Source: CAD feature listing. Evaluate the final solid. Frame: model axes, mm. Face numbers are marked on the shaded views. A direction names the side the tool comes from. Round coordinates to 2 decimals unless told otherwise and drop trailing zeros. Order: outer loops, then holes, each group sorted by start corner. A loop starts at its lowest first (then second) coordinate and runs counter-clockwise, first axis right, second up. Notation, with made-up numbers: (29, -30.75) -> (77, -30.75) arc R12 ccw to (77, -19.75) -> close; hole circle Ø11 at (1, 76.5). An arc over 180 degrees is marked (long way). Answer as CSV lines item,"result".
from build123d import *

# Parameters (mm, degrees)
SKETCH1_W           = 30
SKETCH1_H           = 73
BOSS_EXTRUDE1_DEPTH = 26
SKETCH2_W           = 25
SKETCH2_H           = 16.1
CUT_EXTRUDE1_DEPTH  = 74
SKETCH3_W           = 26
SKETCH3_H           = 24
SKETCH3_H_2         = 16.23422306
CUT_EXTRUDE2_DEPTH  = 5
SKETCH5_W           = 60
SKETCH5_H           = 60
BOSS_EXTRUDE2_DEPTH = 5
FILLET1_R           = 5
SKETCH6_R           = 1.5
CUT_EXTRUDE4_DEPTH  = 5
SKETCH7_R           = 1
CUT_EXTRUDE5_DEPTH  = 4
SKETCH8_W           = 15.5
SKETCH8_H           = 5
CUT_EXTRUDE6_DEPTH  = 42
SKETCH9_W           = 5
SKETCH9_H           = 26
CUT_EXTRUDE7_DEPTH  = 73
SKETCH10_W          = 2
SKETCH10_H          = 8
SKETCH10_H_2        = 7.5
BOSS_EXTRUDE3_DEPTH = 78
SKETCH11_W          = 42
SKETCH11_H          = 0.6
CUT_EXTRUDE8_DEPTH  = 6
SKETCH13_W          = 0.6
SKETCH13_H          = 5
BOSS_EXTRUDE5_DEPTH = 2
SKETCH15_W          = 4
SKETCH15_H          = 16.1
BOSS_EXTRUDE6_DEPTH = 78


with BuildPart() as part:
    # Sketch1 → Boss-Extrude1 (new body)
    with BuildSketch(Plane.XY):
        Rectangle(SKETCH1_W, SKETCH1_H)
    extrude(amount=BOSS_EXTRUDE1_DEPTH)

    # Sketch2 → Cut-Extrude1 (cut, through all)
    with BuildSketch(Plane(origin=(0, 36.5, 0), x_dir=(1, 0, 0), z_dir=(0, 1, 0))):
        with Locations((-0.5, -13.05)):
            Rectangle(SKETCH2_W, SKETCH2_H)
    extrude(amount=-CUT_EXTRUDE1_DEPTH, mode=Mode.SUBTRACT)

    # Sketch3 → Cut-Extrude2 (cut)
    with BuildSketch(Plane.ZY.offset(15)):
        with Locations((13, 21.5)):
            Rectangle(SKETCH3_W, SKETCH3_H)
        with Locations((13, -5.5)):
            Rectangle(SKETCH3_W, SKETCH3_H)
        with Locations((13, -28.61711153)):
            Rectangle(SKETCH3_W, SKETCH3_H_2)
    extrude(amount=-CUT_EXTRUDE2_DEPTH, mode=Mode.SUBTRACT)

    # Sketch5 → Boss-Extrude2 (add)
    with BuildSketch(Plane(origin=(0, -36.5, 0), x_dir=(-1, 0, 0), z_dir=(0, -1, 0))):
        with Locations((0, -13)):
            Rectangle(SKETCH5_W, SKETCH5_H)
    extrude(amount=BOSS_EXTRUDE2_DEPTH)

    # Fillet1
    fillet1_edges = [part.edges().sort_by_distance(p)[0] for p in [
        (30, -39, -17),
        (30, -39, 43),
        (-30, -39, 43),
        (-30, -39, -17),
    ]]
    fillet(fillet1_edges, radius=FILLET1_R)

    # Sketch6 → Cut-Extrude4 (cut)
    with BuildSketch(Plane(origin=(0, -36.5, 0), x_dir=(1, 0, 0), z_dir=(0, 1, 0))):
        with Locations((-24.540514854, 12.671548216)):
            Circle(SKETCH6_R)
        with Locations((24.540514854, 12.671548216)):
            Circle(SKETCH6_R)
        with Locations((-24.540514854, -38.671548216)):
            Circle(SKETCH6_R)
        with Locations((24.540514854, -38.671548216)):
            Circle(SKETCH6_R)
    extrude(amount=-CUT_EXTRUDE4_DEPTH, mode=Mode.SUBTRACT)

    # Sketch7 → Cut-Extrude5 (cut)
    with BuildSketch(Plane(origin=(0, 0, 0), x_dir=(-1, 0, 0), z_dir=(0, 0, -1))):
        with Locations((-7, 31.5)):
            Circle(SKETCH7_R)
        with Locations((-12, 24.5)):
            Circle(SKETCH7_R)
        with Locations((-2, 24.5)):
            Circle(SKETCH7_R)
        with Locations((-7, 18.5)):
            Circle(SKETCH7_R)
    extrude(amount=-CUT_EXTRUDE5_DEPTH, mode=Mode.SUBTRACT)

    # Sketch8 → Cut-Extrude6 (cut)
    with BuildSketch(Plane.ZY.offset(30)):
        with Locations((12.75, -39)):
            Rectangle(SKETCH8_W, SKETCH8_H)
    extrude(amount=-CUT_EXTRUDE6_DEPTH, mode=Mode.SUBTRACT)

    # Sketch9 → Cut-Extrude7 (cut)
    with BuildSketch(Plane(origin=(0, 36.5, 0), x_dir=(1, 0, 0), z_dir=(0, 1, 0))):
        with Locations((-12.5, -13)):
            Rectangle(SKETCH9_W, SKETCH9_H)
    extrude(amount=-CUT_EXTRUDE7_DEPTH, mode=Mode.SUBTRACT)

    # Sketch10 → Boss-Extrude3 (add)
    with BuildSketch(Plane(origin=(0, 36.5, 0), x_dir=(1, 0, 0), z_dir=(0, 1, 0))):
        with Locations((-11, -4)):
            Rectangle(SKETCH10_W, SKETCH10_H)
        with Locations((-11, -22.25)):
            Rectangle(SKETCH10_W, SKETCH10_H_2)
    extrude(amount=-BOSS_EXTRUDE3_DEPTH)

    # Sketch11 → Cut-Extrude8 (cut, through all)
    with BuildSketch(Plane(origin=(0, -36.5, 0), x_dir=(1, 0, 0), z_dir=(0, 1, 0))):
        with Locations((-9, -20.8)):
            Rectangle(SKETCH11_W, SKETCH11_H)
    extrude(amount=-CUT_EXTRUDE8_DEPTH, mode=Mode.SUBTRACT)

    # Sketch13 → Boss-Extrude5 (add)
    with BuildSketch(Plane.ZY.offset(12)):
        with Locations((20.8, -39)):
            Rectangle(SKETCH13_W, SKETCH13_H)
    extrude(amount=-BOSS_EXTRUDE5_DEPTH)

    # Sketch15 → Boss-Extrude6 (add)
    with BuildSketch(Plane(origin=(0, 36.5, 0), x_dir=(1, 0, 0), z_dir=(0, 1, 0))):
        with Locations((4.6, -13.05)):
            Rectangle(SKETCH15_W, SKETCH15_H)
    extrude(amount=-BOSS_EXTRUDE6_DEPTH)


solid = part.part
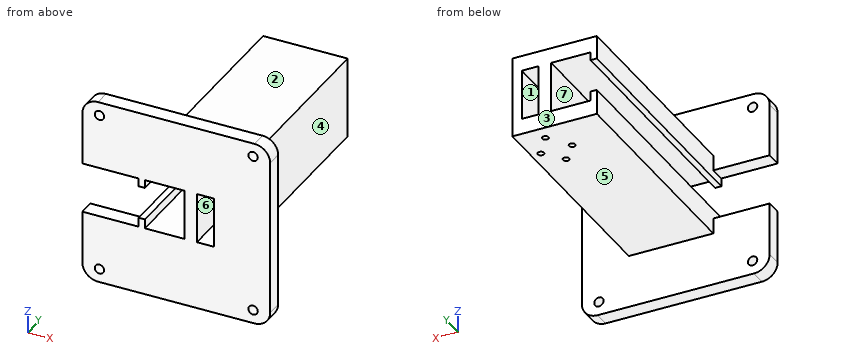
1. Section query C-C on x = -11. Return loops of the section in (y, z).
Results below:
outline,"(-41.5, -17) -> (-36.5, -17) -> (-36.5, 0) -> (36.5, 0) -> (36.5, 8) -> (-41.5, 8) -> close; (-41.5, 18.5) -> (36.5, 18.5) -> (36.5, 26) -> (-36.5, 26) -> (-36.5, 43) -> (-41.5, 43) -> close"
2. Pin query (flat end, axial travel): pin 1 (3 mm diameter, centred on y = -12, z = 26.5, fed in from +X); pin 2 (2 mm diameter, centred on x = 15, y = -17.5, fed in from -Z); pin 3 (5 mm diameter, centred on x = 24.54, z = -12.67, fed in from -Y); pin 4 (1 mm diameter, centred on x = -11, y = 2.5, fed in from +Z). Return the tip coordinate at first contact, or that it passes through.
Results below:
pin 1,"x = 15"
pin 2,"z = 0"
pin 3,"y = -41.5"
pin 4,"z = 26"
3. Section query A-A on z = 16. Return loops of the section in (x, y).
Results below:
outline,"(2.6, -41.5) -> (6.6, -41.5) -> (6.6, 36.5) -> (2.6, 36.5) -> close; (12, -41.5) -> (30, -41.5) -> (30, -36.5) -> (15, -36.5) -> (15, 36.5) -> (12, 36.5) -> close"
4. Reachability of the marked faces 1, 2 and 3 from +Z, -Z, +X, -X, +Y, -Y: full face, straight path, thin tool, end or side. Return the list, or none.
Results below:
face 1,"+Y, -Y"
face 2,"+Z, +X, -X, +Y"
face 3,"+Z, -Z, +X, -X, +Y"
5. Mould query, pull axis Z, two halves, no side actions, for the marked faces 4, 5, 6 and 7. Classes: released by +Z, released by -Z, zero draft, split by the parting line, or undercut.
Results below:
face 4,"zero draft"
face 5,"released by -Z"
face 6,"undercut"
face 7,"undercut"
6. Section query D-D on x = -17.5. Return loops of the section in (y, z), and give its area (4 significant figures).
Results below:
outline,"(-41.5, -17) -> (-36.5, -17) -> (-36.5, 5) -> (-41.5, 5) -> close; (-41.5, 21.1) -> (-36.5, 21.1) -> (-36.5, 43) -> (-41.5, 43) -> close"
area,"219.5 mm2"
7. Section query B-B on y = 18.5. Return loops of the section in (x, z), and give its area (3 significant figures).
Results below:
outline,"(-12, 0) -> (6, 0) -> (6, 4) -> (8, 4) -> (8, 0) -> (15, 0) -> (15, 26) -> (-12, 26) -> (-12, 18.5) -> (-10, 18.5) -> (-10, 21.1) -> (2.6, 21.1) -> (2.6, 5) -> (-10, 5) -> (-10, 8) -> (-12, 8) -> close; hole (6.6, 5) -> (12, 5) -> (12, 21.1) -> (6.6, 21.1) -> close"
area,"383 mm2"
8. Line query: L1, parallel to X at y = -6.5, z = 6; L2, parallel to Z at x = -1, y = -32.5; L3, parallel to Y at x = 7, z = 3. Output: solid intervals per line, ascending. Write a range as [from, to].
Results below:
L1,"[-12, -10], [2.6, 6.6], [12, 15]"
L2,"[0, 5], [21.1, 26]"
L3,"[-41.5, 17.5], [19.5, 30.5], [32.5, 36.5]"
